Autodesk Inventor part; units mm, degrees
ref_plane "YZ Plane" through (0, 0, 0) normal (1, 0, 0) x (0, 1, 0)
ref_plane "XZ Plane" through (0, 0, 0) normal (0, 1, 0) x (-1, 0, 0)
ref_plane "XY Plane" through (0, 0, 0) normal (0, 0, 1) x (1, 0, 0)
sketch "Sketch1" plane through (0, 0, 0) normal (0, 0, 1) x (1, 0, 0)
  line L0 (-15.875, 0) -> (-12.7, 0)
  line L1 (-12.7, 0) -> (-12.7, 22.352)
  line L2 (-9.525, 25.527) -> (9.525, 25.527)
  line L3 (12.7, 22.352) -> (12.7, 0)
  line L4 (12.7, 0) -> (15.875, 0)
  line L5 (15.875, 0) -> (15.875, 25.527)
  line L6 (12.7, 28.702) -> (-12.7, 28.702)
  line L7 (-15.875, 25.527) -> (-15.875, 0)
  arc A0 (-9.525, 25.527) -> (-12.7, 22.352) centre (-9.525, 22.352) ccw
  arc A1 (12.7, 22.352) -> (9.525, 25.527) centre (9.525, 22.352) ccw
  arc A2 (-12.7, 28.702) -> (-15.875, 25.527) centre (-12.7, 25.527) ccw
  arc A3 (15.875, 25.527) -> (12.7, 28.702) centre (12.7, 25.527) ccw
  line L8 (0, 35.2315) -> (0, -5.8719)
  point P0 (0, 0)
  dimension "d0" = 28.702
  dimension "d1" = 31.75
  dimension "d2" = 3.175
  dimension "d3" = 3.175
  dimension "d4" = 3.175
extrude "Extrusion1" add sketch "Sketch1" along normal mid plane 203.2
sketch "Sketch4" plane through (15.875, 0, 101.6) normal (1, 0, 0) x (0, 0, -1)
  line L0 (101.6, -5.7404) -> (101.6, 34.4424) construction
  line L1 (-40.64, 0) -> (243.84, 0) construction
  circle A0 centre (114.3, 12.7) radius 3.175
  point P0 (101.6, 0)
  dimension "d34" = 12.7
  dimension "d35" = 12.7
  dimension "d36" = 6.35
extrude "Extrusion4" cut sketch "Sketch4" against normal up to surface (31.75 mm away)
pattern_linear "Rectangular Pattern3" count 15 spacing 25.4 along (0, 0, 1) count 15 spacing 25.4 along (0, 0, -1) of "Extrusion4"
equation "\"d5\" = Support2Length"
equation "\"Support2Length\" = 203.2"
properties part number "NSupportChannel2" material "Aluminum 6061"
Here's how the part is built. I have some questions about the finished solid (model axes, mm). A direction names the side the tool comes from. Give positions to 0.01 mm unless a question says otherwise; leave off trailing zeros. Write each loop counter-clockwise with the first axis right and the second up, starting at its lowest first coordinate (ties: lowest second). Pieces come first, ordered by that corner, then holes. Notation, with made-up numbers: M -15,26 L 10,26 A22 cw 10,44 Z; hole C -36,5.25 d11. An arc over 180 degrees is marked long. Put each result on its own line as item: value. Start each with the question number.
Item 1: Thinking about a two-plate mould opening in Y: for faces 3 (the cylindrical face through (-11.795, 24.572, -1.422)), 4 (the flat face through (-1, 26, -101.6)), 5 (the cylindrical face through (-14.27, 10.77, -86.38)), which applies, +Y half, -Y half, draft (parallel to the pull), parting line (faces both ways), or undercut?
Item 2: Will these pins go through, and if not, where does the flat tip stop? pin 1 (4 mm diameter, centred on y = 12.7, z = 38.1, fed in from -X); pin 2 (9.5 mm diameter, centred on x = 2, z = 30, fed in from -Y).
Item 3: On a 3-axis mill with a long thin cutter (end or side, diameter ignored), from which of +Z, -Z, +X, -X, +Y, -Y can I reach the whole of each face in a straight line? I mean faces 1 (the flat face through (0, 25.527, -1)), 2 (the cylindrical face through (14.3, 9.9, 11.2)). Say none if no direction works.
Item 4: If we section it at C-C, the plane z = 1: Write out the boundary of the cut face in (x, y) (3 decimals).
Item 5: I need wall thicknesses on L1, parallel to X at y = 7.75, z = 35.5 (3 decimals); L2, parallel to Y at x = 2, z = 5; L3, parallel to Y at x = 14.85, z = -38.1 (3 decimals). Which ranges of each line are inside material? Lowest first, please. Write a range as from..to.
Item 6: If we section it at A-A, the plane y = 7: Write out the boundary of the cut face in (x, z) (3 decimals), then the cut area to 3 significant figures.
Item 7: If we section it at B-B, the plane z = 88.9: Write out the boundary of the cut face in (x, y) (3 decimals), then the cut area to 3 significant figures.
Values:
1. face 3: -Y half
1. face 4: draft
1. face 5: undercut
2. pin 1: through
2. pin 2: y = 25.53
3. face 1: +Z, -Z, -Y
3. face 2: +X, -X
4. outline: M -15.875,0 L -12.7,0 L -12.7,22.352 A3.175 cw -9.525,25.527 L 9.525,25.527 A3.175 cw 12.7,22.352 L 12.7,0 L 15.875,0 L 15.875,25.527 A3.175 ccw 12.7,28.702 L -12.7,28.702 A3.175 ccw -15.875,25.527 Z
5. L1: -15.875..-12.7, 12.7..15.875
5. L2: 25.53..28.7
5. L3: 0..9.525, 15.875..27.863
6. outline: M -15.875,-101.6 L -12.7,-101.6 L -12.7,101.6 L -15.875,101.6 Z; M 12.7,-101.6 L 15.875,-101.6 L 15.875,101.6 L 12.7,101.6 Z
6. area: 1,290 mm²
7. outline: M -15.875,0 L -12.7,0 L -12.7,9.525 L -15.875,9.525 Z; M -15.875,15.875 L -12.7,15.875 L -12.7,22.352 A3.175 cw -9.525,25.527 L 9.525,25.527 A3.175 cw 12.7,22.352 L 12.7,15.875 L 15.875,15.875 L 15.875,25.527 A3.175 ccw 12.7,28.702 L -12.7,28.702 A3.175 ccw -15.875,25.527 Z; M 12.7,0 L 15.875,0 L 15.875,9.525 L 12.7,9.525 Z
7. area: 223 mm²
